```python
from build123d import *

# Parameters (mm, degrees)
BOSS_EXTRUDE1_DEPTH = 16
BOSS_EXTRUDE2_START = -2
BOSS_EXTRUDE2_DEPTH = 2
CHAMFER2_SIZE       = 2.5


with BuildPart() as part:
    # Sketch2 → Boss-Extrude1 (new, symmetric)
    with BuildSketch(Plane(origin=(0, 0, 0), x_dir=(1, 0, 0), z_dir=(0, 1, 0))):
        with BuildLine():
            Line((-58.637924155, 125.749434155), (-59.166556644, 126.883090185))
            ThreePointArc((-59.166556644, 126.883090185), (-2.609123321, 139.975685301), (54.396940678, 128.999894748))
            Line((54.396940678, 128.999894748), (53.971953665, 127.832252528))
            ThreePointArc((53.971953665, 127.832252528), (56.314568974, 126.8124168), (58.637924155, 125.749434155))
            Line((58.637924155, 125.749434155), (58.110010989, 124.617320718))
            ThreePointArc((58.110010989, 124.617320718), (2.5, 137.477270849), (-53.540801289, 126.647671109))
            Line((-53.540801289, 126.647671109), (-53.971953665, 127.832252528))
            ThreePointArc((-53.971953665, 127.832252528), (-56.314568974, 126.8124168), (-58.637924155, 125.749434155))
        make_face()
    extrude(amount=BOSS_EXTRUDE1_DEPTH, both=True)

    # Sketch3 → Boss-Extrude2 (add)
    with BuildSketch(Plane.XZ.offset(16).offset(BOSS_EXTRUDE2_START)):
        with BuildLine():
            Line((49.470958786, -133.637099029), (48.718270464, -131.249876659))
            ThreePointArc((48.718270464, -131.249876659), (-2.609123321, -139.975685301), (-53.575680531, -129.343134552))
            Line((-53.575680531, -129.343134552), (-58.637924155, -125.749434155))
            Line((-58.637924155, -125.749434155), (-54.532389112, -131.652833383))
            ThreePointArc((-54.532389112, -131.652833383), (-2.718243325, -142.474071863), (49.470958786, -133.637099029))
        make_face()
        with BuildLine():
            Line((52.61897195, -127.033435721), (58.637924155, -125.749434155))
            Line((58.637924155, -125.749434155), (51.662263369, -124.723736889))
            ThreePointArc((51.662263369, -124.723736889), (2.390873136, -134.978826953), (-47.212790972, -126.475105727))
            Line((-47.212790972, -126.475105727), (-47.965548485, -128.86254754))
            ThreePointArc((-47.965548485, -128.86254754), (2.5, -137.477270849), (52.61897195, -127.033435721))
        make_face()
    extrude(amount=BOSS_EXTRUDE2_DEPTH)

    # Chamfer2
    chamfer2_edges = [part.edges().sort_by_distance(p)[0] for p in [
        (-4.601256001, -14, -139.924366867),
        (4.540431296, -14, -137.425014039),
    ]]
    chamfer(chamfer2_edges, length=CHAMFER2_SIZE - 0.0001)  # a hair under: the kernel refuses the full size


solid = part.part
```
Check sheet for the modelled part. Datum: model origin and axes. Units: mm. A direction names the side the tool comes from. Give positions to 0.01 mm unless a question says otherwise; leave off trailing zeros. Write each loop counter-clockwise with the first axis right and the second up, starting at its lowest first coordinate (ties: lowest second). Pieces come first, ordered by that corner, then holes. Notation, with made-up numbers: (7.25, -6.5) - (62.25, -6.5) arc R28 ccw to (62.25, 14.5) - close; hole circle Ø6 at (-31.5, 16). An arc over 180 degrees is marked (long way). Answer as a JSON object with one key per item and string values. Group by question number.
1) Depth check by flat-ended pin: P1, Ø4, axis at x = -46, y = -1, coming from the -Z side; P2, Ø5, axis at y = -9.5, z = -127.5, coming from the +X side; P3, Ø1, axis at x = -15.5, y = 5.5, coming from the +Z side. Enter the tip coordinate at first touch or a pass-through.
2) Sectioned sample at B-B (y = -12.5). Record the cut outline in (x, z), then the cut area to 3 significant figures.
3) Release check for a two-part mould opening along Z. For faces 1 (the face through (0, 16, -138)), 2 (the face through (49.016, -14.219, -132.195)), 3 (the face through (3.3, 3.78, -137.46)) record: pulls with the +Z half, pulls with the -Z half, needs draft (parallel to the pull), parting line crosses it, or undercut.
4) Sectioned sample at A-A (y = -3.5). Record the cut outline in (x, z), then the cut area to 3 significant figures.
5) Access from +Z, -Z, +X, -X, +Y, -Y to the whole of each face (thin tool, end or side, straight path). Record for faces 4 (the face through (-56.28, 0.22, -126.83)), 5 (the face through (-1.1, -16, -135.4)).
6) Thickness scan on probe 1 along Z at (x, y) = (1, 12); probe 2 along Y at (x, z) = (-50, -131.5); probe 3 along Z at (x, y) = (41.5, 9.5). Record the ranges inside material, lowest first. Write a range as from..to.
Geometry results:
{
 "1": {"P1": "stops at z = -132.91", "P2": "stops at x = 58.64", "P3": "stops at z = -136.57"},
 "2": {"outline": "(-59.17, -126.88) arc R140 ccw to (-57.24, -127.77) - (-56.14, -129.34) arc R141 ccw to (49.02, -132.2) - (48.72, -131.25) arc R140 ccw to (54.4, -129) - (53.97, -127.83) arc R138.16 ccw to (58.64, -125.75) - (58.11, -124.62) arc R137.5 cw to (56.37, -125.42) - (54.51, -125.14) arc R136.5 cw to (-47.66, -127.91) - (-47.97, -128.86) arc R137.5 cw to (-53.54, -126.65) - (-53.97, -127.83) arc R138.16 cw to (-58.64, -125.75) - close", "area": "504 mm^2"},
 "3": {"face 1": "needs draft", "face 2": "undercut", "face 3": "pulls with the +Z half"},
 "4": {"outline": "(-59.17, -126.88) arc R140 ccw to (54.4, -129) - (53.97, -127.83) arc R138.16 ccw to (58.64, -125.75) - (58.11, -124.62) arc R137.5 cw to (-53.54, -126.65) - (-53.97, -127.83) arc R138.16 cw to (-58.64, -125.75) - close", "area": "290 mm^2"},
 "5": {"face 4": "+Z, +Y, -Y", "face 5": "+Z, -Z, +X, -X, -Y"},
 "6": {"probe 1": "z = -140..-137.5", "probe 2": "y = -16..-12.19", "probe 3": "z = -133.71..-131.09"}
}
